```python
from build123d import *

# Parameters (mm, degrees)
SKETCH1_W              = 127
SKETCH1_H              = 50.8
BOSS_EXTRUDE1_DEPTH    = 1.5875
SKETCH2_R              = 1.27
CUT_EXTRUDE1_DEPTH     = 69.410015029
F_10_CLEARANCE_HOLE1_D = 5.6134


with BuildPart() as part:
    # Sketch1 → Boss-Extrude1 (new body)
    with BuildSketch(Plane(origin=(0, 0, 0), x_dir=(1, 0, 0), z_dir=(0, 1, 0))):
        Rectangle(SKETCH1_W, SKETCH1_H)
    extrude(amount=BOSS_EXTRUDE1_DEPTH)

    # Sketch2 → Cut-Extrude1 (cut, through all)
    with BuildSketch(Plane(origin=(0, 1.5875, 0), x_dir=(1, 0, 0), z_dir=(0, 1, 0))):
        with Locations(Location((-12.7, 0, 0), (0, 0, 270))):
            Circle(SKETCH2_R)
        with Locations(Location((12.7, 0, 0), (0, 0, 270))):
            Circle(SKETCH2_R)
        with BuildLine():
            Line((-57.15, 16.66875), (-44.45, 16.66875))
            ThreePointArc((-44.45, 16.66875), (-42.06875, 19.05), (-44.45, 21.43125))
            Line((-44.45, 21.43125), (-57.15, 21.43125))
            ThreePointArc((-57.15, 21.43125), (-59.53125, 19.05), (-57.15, 16.66875))
        make_face()
        with BuildLine():
            Line((-57.15, -21.43125), (-44.45, -21.43125))
            ThreePointArc((-44.45, -21.43125), (-42.06875, -19.05), (-44.45, -16.66875))
            Line((-44.45, -16.66875), (-57.15, -16.66875))
            ThreePointArc((-57.15, -16.66875), (-59.53125, -19.05), (-57.15, -21.43125))
        make_face()
        with BuildLine():
            Line((44.45, 16.66875), (57.15, 16.66875))
            ThreePointArc((57.15, 16.66875), (59.53125, 19.05), (57.15, 21.43125))
            Line((57.15, 21.43125), (44.45, 21.43125))
            ThreePointArc((44.45, 21.43125), (42.06875, 19.05), (44.45, 16.66875))
        make_face()
        with BuildLine():
            Line((44.45, -21.43125), (57.15, -21.43125))
            ThreePointArc((57.15, -21.43125), (59.53125, -19.05), (57.15, -16.66875))
            Line((57.15, -16.66875), (44.45, -16.66875))
            ThreePointArc((44.45, -16.66875), (42.06875, -19.05), (44.45, -21.43125))
        make_face()
    extrude(amount=-CUT_EXTRUDE1_DEPTH, mode=Mode.SUBTRACT)

    # #10 Clearance Hole1 (through all)
    with Locations(Plane(origin=(0, 1.5875, 0), x_dir=(1, 0, 0), z_dir=(0, 1, 0))):
        with Locations((-12.7, 0), (12.7, 0)):
            Hole(F_10_CLEARANCE_HOLE1_D / 2)


solid = part.part
```
The listing builds one solid part. Answer for the finished solid, in the listing's coordinates (mm). A direction names the side the tool comes from. Round coordinates to 2 decimals unless told otherwise and drop trailing zeros. Write each loop counter-clockwise with the first axis right and the second up, starting at its lowest first coordinate (ties: lowest second). Pieces come first, ordered by that corner, then holes. Notation, with made-up numbers: (-27, 16.25) -> (19, 16.25) arc R24 cw to (19, 49.25) -> close; hole circle Ø6 at (19, 6.25). An arc over 180 degrees is marked (long way). Use CSV: the item, a comma, the result in double quotes. Start each with the question number.
(1) Section B-B on z = 0 is taken. Give the vertices of the cut face in (x, y), then the cut area to 3 significant figures.
(2) Section C-C on x = -46 is taken. Give the vertices of the cut face in (y, z).
(3) Consider L1, parallel to Z at x = -53, y = 0.55; L2, parallel to Z at x = 12.7, y = 0.8; L3, parallel to X at y = 1.45, z = 1. Determine where each line is inside the solid, lowest interval first. Write a range as from..to.
(4) Which of the six approach directions +Z, -Z, +X, -X, +Y, -Y give full straight-line access (tool end or side, diameter ignored) to faces 1 (the face through (-1, 0, 0)), 2 (the face through (-59.53, 0.8, 19))?
(5) Section A-A on x = 12.7 is taken. Give the vertices of the cut face in (y, z), then the cut area to 3 significant figures.
(6) Section D-D on y = 0.75 is taken. Give the vertices of the cut face in (x, z), then the cut area to 3 significant figures.
(7) This flat-tipped pin is pushed along its axis until it touches: pin 1 (4.5 mm diameter, centred on x = -12.7, z = 0, fed in from -Y). Where does it stop, or does it pass through?
(8) The mould has two halves that part along Z. Classify faces 3 (the face through (-42.07, 0.8, -19)), 4 (the face through (-1, 1.588, 0)): released by +Z, released by -Z, zero draft, split by the parting line, or undercut.
A:
1,outline,"(-63.5, 0) -> (-15.51, 0) -> (-15.51, 1.59) -> (-63.5, 1.59) -> close; (-9.89, 0) -> (9.89, 0) -> (9.89, 1.59) -> (-9.89, 1.59) -> close; (15.51, 0) -> (63.5, 0) -> (63.5, 1.59) -> (15.51, 1.59) -> close"
1,area,"184 mm²"
2,outline,"(0, -25.4) -> (1.59, -25.4) -> (1.59, -21.43) -> (0, -21.43) -> close; (0, -16.67) -> (1.59, -16.67) -> (1.59, 16.67) -> (0, 16.67) -> close; (0, 21.43) -> (1.59, 21.43) -> (1.59, 25.4) -> (0, 25.4) -> close"
3,L1,"z = -25.4..-21.43, -16.67..16.67, 21.43..25.4"
3,L2,"z = -25.4..-2.81, 2.81..25.4"
3,L3,"x = -63.5..-15.32, -10.08..10.08, 15.32..63.5"
4,face 1,"+Z, -Z, +X, -X, -Y"
4,face 2,"+Y, -Y"
5,outline,"(0, -25.4) -> (1.59, -25.4) -> (1.59, -2.81) -> (0, -2.81) -> close; (0, 2.81) -> (1.59, 2.81) -> (1.59, 25.4) -> (0, 25.4) -> close"
5,area,"71.7 mm²"
6,outline,"(-63.5, -25.4) -> (63.5, -25.4) -> (63.5, 25.4) -> (-63.5, 25.4) -> close; hole (-57.15, -21.43) -> (-44.45, -21.43) arc R2.38 ccw to (-44.45, -16.67) -> (-57.15, -16.67) arc R2.38 ccw to start; hole (-57.15, 16.67) -> (-44.45, 16.67) arc R2.38 ccw to (-44.45, 21.43) -> (-57.15, 21.43) arc R2.38 ccw to start; hole circle Ø5.61 at (-12.7, 0); hole circle Ø5.61 at (12.7, 0); hole (44.45, -21.43) -> (57.15, -21.43) arc R2.38 ccw to (57.15, -16.67) -> (44.45, -16.67) arc R2.38 ccw to start; hole (44.45, 16.67) -> (57.15, 16.67) arc R2.38 ccw to (57.15, 21.43) -> (44.45, 21.43) arc R2.38 ccw to start"
6,area,"6,090 mm²"
7,pin 1,"passes through"
8,face 3,"undercut"
8,face 4,"zero draft"
